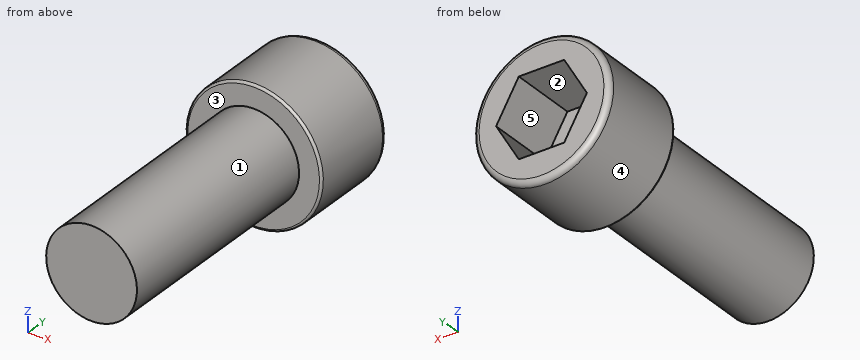
from build123d import *

# Parameters (mm, degrees)
SKETCH1_R           = 3
BOSS_EXTRUDE1_DEPTH = 4
FILLET1_R           = 0.25
CUT_EXTRUDE1_DEPTH  = 3
FILLET2_R           = 0.1
SKETCH3_R           = 2
BOSS_EXTRUDE2_DEPTH = 10


with BuildPart() as part:
    # Sketch1 → Boss-Extrude1 (new body)
    with BuildSketch(Plane(origin=(0, 0, 0), x_dir=(1, 0, 0), z_dir=(0, 1, 0))):
        with Locations(Location((0, 0, 0), (0, 0, 270))):
            Circle(SKETCH1_R)
    extrude(amount=BOSS_EXTRUDE1_DEPTH)

    # Fillet1
    fillet1_edges = [part.edges().sort_by_distance(p)[0] for p in [
        (0, 4, -3),
    ]]
    fillet(fillet1_edges, radius=FILLET1_R)

    # Sketch2 → Cut-Extrude1 (cut)
    with BuildSketch(Plane(origin=(0, 4, 0), x_dir=(1, 0, 0), z_dir=(0, 1, 0))):
        Polygon((2, 0), (1, 1.732050808), (-1, 1.732050808), (-2, 0), (-1, -1.732050808), (1, -1.732050808), align=None)
    extrude(amount=-CUT_EXTRUDE1_DEPTH, mode=Mode.SUBTRACT)

    # Fillet2
    fillet2_edges = [part.edges().sort_by_distance(p)[0] for p in [
        (0, 0, -3),
    ]]
    fillet(fillet2_edges, radius=FILLET2_R)

    # Sketch3 → Boss-Extrude2 (add)
    with BuildSketch(Plane.XZ):
        with Locations(Location((0, 0, 0), (0, 0, 90))):
            Circle(SKETCH3_R)
    extrude(amount=BOSS_EXTRUDE2_DEPTH)


solid = part.part
For this review, take the finished solid that the model builds, in its own axes (mm). Face numbers are marked on the shaded views. A direction names the side the tool comes from. Round coordinates to 2 decimals unless told otherwise and drop trailing zeros. Loops run counter-clockwise (first coordinate to the right, second up) from the corner with the lowest first, then second, coordinate; pieces in that order, holes last. Notation, with made-up numbers: (-28.75, 72) - (19.25, 72) arc R32 cw to (19.25, 110) - close; hole circle Ø3 at (83, -39). An arc over 180 degrees is marked (long way). Put each result on its own line as item: value. Start each with the question number.
1. Consider section B-B on y = -7.5. State the section outline as (x, z) points, plus the area to 3 significant figures.
2. For the marked faces 4 and 5, list the 3-axis set-ups (+Z, -Z, +X, -X, +Y, -Y) from which the entire face can be reached by the end or side of a thin tool; tool diameter is ignored.
3. Consider section A-A on y = 2.25. State the section outline as (x, z) points, plus the area to 3 significant figures.
4. For probe 1 along Y at (x, z) = (0, 2.5); probe 2 along Y at (x, z) = (1.5, 0.5); probe 3 along X at (y, z) = (-9.25, 0), list the stretches that pass through material, from the lowest coordinate up. Write a range as [from, to].
5. Mouldability with a two-part tool opening along Z and no side actions: class the marked faces 1, 2 and 3 as +Z half, -Z half, draft (parallel to the pull), parting line (faces both ways), or undercut.
6. Insertion check: P1, Ø1.5, axis at x = 2.5, y = 0.5, coming from the +Z side; P2, Ø1.5, axis at y = -6, z = -1, coming from the +X side. Each pin has a flat end and moves straight along its axis. Give the tip position at first contact, or say it passes through.
Result sheet:
1. outline: circle Ø4 at (0, 0)
1. area: 12.6 mm^2
2. face 4: +Y, -Y
2. face 5: +Y
3. outline: circle Ø6 at (0, 0); hole (-2, 0) - (-1, -1.73) - (1, -1.73) - (2, 0) - (1, 1.73) - (-1, 1.73) - close
3. area: 17.9 mm^2
4. probe 1: [0, 4]
4. probe 2: [-10, 1]
4. probe 3: [-2, 2]
5. face 1: parting line
5. face 2: undercut
5. face 3: draft
6. P1: z = 2.44
6. P2: x = 1.98
